```python
from build123d import *

# Parameters (mm, degrees)
SKETCH_R         = 8.25
EXTRUDE_DEPTH    = 1.6
CHAMFER_SIZE     = 1
SKETCH001_W      = 15
SKETCH001_H      = 4.2
EXTRUDE001_DEPTH = 17.4


with BuildPart() as chamfer_body:
    # Sketch → Extrude (new body)
    with BuildSketch(Plane.XY):
        Circle(SKETCH_R)
    extrude(amount=EXTRUDE_DEPTH)

    # Chamfer
    chamfer_edges = [chamfer_body.edges().sort_by_distance(p)[0] for p in [
        (-8.25, 0, 1.6),
    ]]
    chamfer(chamfer_edges, length=CHAMFER_SIZE)


with BuildPart() as fusion:
    # Sketch001 (on Face3 of Chamfer) → Extrude001 (new body)
    with BuildSketch(Plane(origin=(0, 0, 0), x_dir=(1, 0, 0), z_dir=(0, 0, -1))):
        Rectangle(SKETCH001_W, SKETCH001_H)
    extrude(amount=EXTRUDE001_DEPTH)

    # Fusion: union Chamfer body
    add(chamfer_body.part)


solid = fusion.part
```
Geometry check sheet. Reference: the model listing, model coordinates, mm. A direction names the side the tool comes from. Give positions to 0.01 mm unless a question says otherwise; leave off trailing zeros. Order: outer loops, then holes, each group sorted by start corner. A loop starts at its lowest first (then second) coordinate and runs counter-clockwise, first axis right, second up.
1. Thickness scan on L1, parallel to Z at x = -1, y = -5; L2, parallel to Y at x = 4.25, z = -15.25; L3, parallel to X at y = -0.75, z = -12.75. Record the ranges inside material, lowest first.
2. Section check A-A, the plane y = 0. Enter the section's corners in (x, z).
3. Gauge pin test, flat ends, axial feed: pin 1 Ø5 at (x, z) = (3.5, -9) entering from -Y; pin 2 Ø4 at (x, z) = (3, -4) entering from +Y; pin 3 Ø3.5 at (y, z) = (0.5, -11) entering from -X. Record the tip position at first contact, or that the pin passes through.
4. Section check C-C, the plane z = -6. Enter the section's corners in (x, y), and give its area (3 significant figures).
5. Section check B-B, the plane x = 0. Enter the section's corners in (y, z), and give its area (3 significant figures).
6. Access from +Z, -Z, +X, -X, +Y, -Y to the whole of each face (thin tool, end or side, straight path). Record for faces 1 (the face through (7.5, 0, -9)), 2 (the face through (-7.5, 0, -9)), 3 (the face through (0, 2.1, -9)), 4 (the face through (0, 0, -17.4)), 5 (the face through (0, -2.1, -9)).
Values follow:
1. L1: z = 0 to 1.6
1. L2: y = -2.1 to 2.1
1. L3: x = -7.5 to 7.5
2. outline: (-8.25, 0) - (-7.5, 0) - (-7.5, -17.4) - (7.5, -17.4) - (7.5, 0) - (8.25, 0) - (8.25, 0.6) - (7.25, 1.6) - (-7.25, 1.6) - (-8.25, 0.6) - close
3. pin 1: stops at y = -2.1
3. pin 2: stops at y = 2.1
3. pin 3: stops at x = -7.5
4. outline: (-7.5, -2.1) - (7.5, -2.1) - (7.5, 2.1) - (-7.5, 2.1) - close
4. area: 63.0 mm2
5. outline: (-8.25, 0) - (-2.1, 0) - (-2.1, -17.4) - (2.1, -17.4) - (2.1, 0) - (8.25, 0) - (8.25, 0.6) - (7.25, 1.6) - (-7.25, 1.6) - (-8.25, 0.6) - close
5. area: 98.5 mm2
6. face 1: -Z, +X, +Y, -Y
6. face 2: -Z, -X, +Y, -Y
6. face 3: -Z, +X, -X, +Y
6. face 4: -Z, +X, -X, +Y, -Y
6. face 5: -Z, +X, -X, -Y
